from build123d import *
from OCP.BRepFilletAPI import BRepFilletAPI_MakeChamfer

# Parameters (mm, degrees)
BOSS_EXTRUDE1_DEPTH = 15
CUT_EXTRUDE4_DEPTH  = 5
SKETCH7_R           = 3.1
CUT_EXTRUDE6_DEPTH  = 66.86721491
FILLET1_R           = 7.5
CUT_EXTRUDE7_DEPTH  = 5
CUT_EXTRUDE8_DEPTH  = 5
FILLET2_R           = 1.5
BOSS_EXTRUDE2_DEPTH = 5
SKETCH6_R           = 3.1
CUT_EXTRUDE5_DEPTH  = 66.86721491
CHAMFER8_SIZE       = 15
CHAMFER8_SIZE_2     = 5


with BuildPart() as part:
    # Sketch1 → Boss-Extrude1 (new body)
    with BuildSketch(Plane(origin=(0, 0, 0), x_dir=(1, 0, 0), z_dir=(0, 1, 0))):
        Polygon((0, 0), (-35, 0), (-45, 12.85), (-45, 32.85), (-35, 45.7), (0, 45.7), (0, 40.7), (-22.5, 40.7), (-22.5, 35.5), (0, 35.5), (0, 27.85), (-22.5, 27.85), (-22.5, 17.85), (0, 17.85), (0, 10.2), (-22.5, 10.2), (-22.5, 5), (0, 5), align=None)
    extrude(amount=BOSS_EXTRUDE1_DEPTH)

    # Sketch5 → Cut-Extrude4 (cut)
    with BuildSketch(Plane(origin=(0, 15, 0), x_dir=(1, 0, 0), z_dir=(0, 1, 0))):
        Polygon((-41.639528096, 22.85), (-38.319764048, 17.1), (-31.680235952, 17.1), (-28.360471904, 22.85), (-31.680235952, 28.6), (-38.319764048, 28.6), align=None)
    extrude(amount=-CUT_EXTRUDE4_DEPTH, mode=Mode.SUBTRACT)

    # Sketch7 → Cut-Extrude6 (cut, through all)
    with BuildSketch(Plane.XY):
        with Locations((-7.5, 7.5)):
            Circle(SKETCH7_R)
    extrude(amount=-CUT_EXTRUDE6_DEPTH, mode=Mode.SUBTRACT)

    # Fillet1
    fillet1_edges = [part.edges().sort_by_distance(p)[0] for p in [
        (0, 0, -43.2),
        (0, 0, -31.675),
        (0, 0, -2.5),
        (0, 15, -43.2),
        (0, 15, -31.675),
        (0, 15, -2.5),
        (0, 0, -14.025),
        (0, 15, -14.025),
    ]]
    fillet(fillet1_edges, radius=FILLET1_R - 0.0001)  # a hair under: the kernel refuses the full size

    # Sketch8 → Cut-Extrude7 (cut)
    with BuildSketch(Plane.XY.offset(-27.85)):
        Polygon((-9.839641819, 13.713647036), (-14.050997093, 8.580634267), (-11.711355274, 2.366987231), (-5.160358181, 1.286352964), (-0.949002907, 6.419365733), (-3.288644726, 12.633012769), align=None)
    extrude(amount=-CUT_EXTRUDE7_DEPTH, mode=Mode.SUBTRACT)

    # Sketch9 → Cut-Extrude8 (cut)
    with BuildSketch(Plane(origin=(0, 0, -17.85), x_dir=(-1, 0, 0), z_dir=(0, 0, -1))):
        Polygon((9.839641819, 13.713647036), (3.288644726, 12.633012769), (0.949002907, 6.419365733), (5.160358181, 1.286352964), (11.711355274, 2.366987231), (14.050997093, 8.580634267), align=None)
    extrude(amount=-CUT_EXTRUDE8_DEPTH, mode=Mode.SUBTRACT)

    # Fillet2
    fillet2_edges = [part.edges().sort_by_distance(p)[0] for p in [
        (-22.5, 7.5, -40.7),
        (-22.5, 7.5, -35.5),
        (-22.5, 7.5, -27.85),
        (-22.5, 7.5, -17.85),
        (-22.5, 7.5, -10.2),
        (-22.5, 7.5, -5),
    ]]
    fillet(fillet2_edges, radius=FILLET2_R)

    # Sketch15 → Boss-Extrude2 (add)
    with BuildSketch(Plane.XZ):
        Polygon((-35, 0), (-45, -12.85), (-45, -32.85), (-35, -45.7), (-22.5, -45.7), (-22.5, 0), align=None)
    extrude(amount=BOSS_EXTRUDE2_DEPTH)

    # Sketch6 → Cut-Extrude5 (cut, through all)
    with BuildSketch(Plane(origin=(0, 10, 0), x_dir=(1, 0, 0), z_dir=(0, 1, 0))):
        with Locations(Location((-35, 22.85, 0), (0, 0, 270))):
            Circle(SKETCH6_R)
    extrude(amount=-CUT_EXTRUDE5_DEPTH, mode=Mode.SUBTRACT)

    # Chamfer8
    chamfer8_edges_1 = [part.edges().sort_by_distance(p)[0] for p in [
        (-22.5, 0, -3.25),
    ]]
    chamfer8_side_1 = [part.faces().sort_by_distance(p)[0] for p in [
        (-22.4, 0, -3.25),
    ]]
    chamfer8_edges_2 = [part.edges().sort_by_distance(p)[0] for p in [
        (-22.5, 0, -42.45),
    ]]
    chamfer8_side_2 = [part.faces().sort_by_distance(p)[0] for p in [
        (-22.5, -0.1, -42.45),
    ]]
    chamfer8_edges_3 = [part.edges().sort_by_distance(p)[0] for p in [
        (-22.5, 0, -14.025),
    ]]
    chamfer8_side_3 = [part.faces().sort_by_distance(p)[0] for p in [
        (-22.5, -0.1, -14.025),
    ]]
    chamfer8_edges_4 = [part.edges().sort_by_distance(p)[0] for p in [
        (-22.5, 0, -31.675),
    ]]
    chamfer8_side_4 = [part.faces().sort_by_distance(p)[0] for p in [
        (-22.5, -0.1, -31.675),
    ]]
    chamfer8 = BRepFilletAPI_MakeChamfer(part.part.solid().wrapped)
    for e in chamfer8_edges_1:
        chamfer8.Add(CHAMFER8_SIZE - 0.0001, CHAMFER8_SIZE_2 - 0.0001, e.wrapped, chamfer8_side_1[0].wrapped)
    for e in chamfer8_edges_2:
        chamfer8.Add(CHAMFER8_SIZE_2 - 0.0001, CHAMFER8_SIZE - 0.0001, e.wrapped, chamfer8_side_2[0].wrapped)
    for e in chamfer8_edges_3:
        chamfer8.Add(CHAMFER8_SIZE_2 - 0.0001, CHAMFER8_SIZE - 0.0001, e.wrapped, chamfer8_side_3[0].wrapped)
    for e in chamfer8_edges_4:
        chamfer8.Add(CHAMFER8_SIZE_2 - 0.0001, CHAMFER8_SIZE - 0.0001, e.wrapped, chamfer8_side_4[0].wrapped)
    add(Compound.cast(chamfer8.Shape()), mode=Mode.REPLACE)  # a hair under: the kernel refuses the full size


solid = part.part
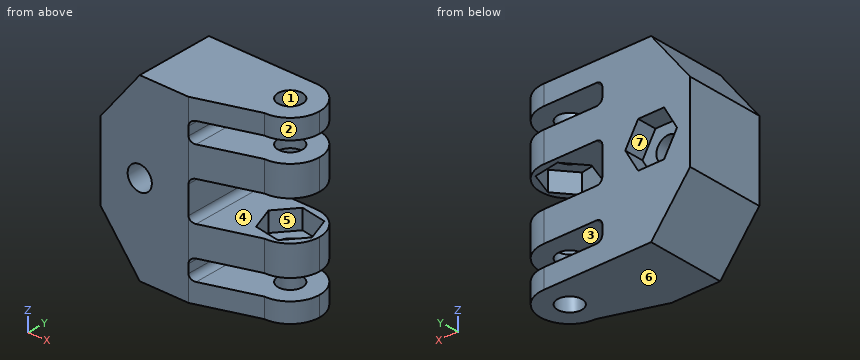
Read the model definition and answer for the solid it produces. Units are mm, in the model's axes. Face numbers are marked on the shaded views. A direction names the side the tool comes from. Coordinates: 2 decimals unless noted, no trailing zeros. Order: outer loops, then holes, each group sorted by start corner. A loop starts at its lowest first (then second) coordinate and runs counter-clockwise, first axis right, second up. Notation, with made-up numbers: M 30,-19 L 72,-19 A24 cw 72,-8 Z; hole C 23.5,80 d10. An arc over 180 degrees is marked long. Put each result on its own line as item: value. Start each with the question number.
Item 1: Section B-B, the plane x = -20 is taken. Determine the outline of the cut face in (y, z).
Item 2: Section C-C, the plane z = -23.5 is taken. Determine the outline of the cut face in (x, y).
Item 3: Consider probe 1 along Z at (x, y) = (-19.5, 13.75); probe 2 along Z at (x, y) = (-4, 3.75); probe 3 along Y at (x, z) = (-7.5, -2.4). Determine where each line is inside the solid, lowest interval first. Write a range as [from, to].
Item 4: Given pin 1 Ø10 at (x, y) = (-7.5, 7.5) entering from +Z; pin 2 Ø3 at (x, y) = (-40.5, 7.5) entering from -Z; pin 3 Ø5 at (y, z) = (-0.5, -24.5) entering from +X; pin 4 Ø10 at (y, z) = (1, -17.5) entering from +X, each flat-ended and moving along its own axis, determine where each tip first touches the part or whether it passes through.
Item 5: The mould has two halves that part along X. Classify the marked faces 1, 2 and 3: +X half, -X half, draft (parallel to the pull), parting line (faces both ways), or undercut.
Item 6: For the marked faces 4, 5, 6 and 7, determine the directions among +Z, -Z, +X, -X, +Y, -Y from which every point of the face is accessible in a straight line to the end or side of a thin tool.
Computed:
1. outline: M -4.17,-45.7 L 15,-45.7 L 15,-40.7 L -4.17,-40.7 Z; M -4.17,-35.5 L 15,-35.5 L 15,-27.85 L -4.17,-27.85 Z; M -4.17,-17.85 L 15,-17.85 L 15,-10.2 L -4.17,-10.2 Z; M -4.17,-5 L 15,-5 L 15,0 L -4.17,0 Z
2. outline: M -45,-5 L -38.03,-5 L -38.03,10 L -41.26,10 L -41.26,15 L -45,15 Z; M -31.97,-5 L -22.5,-5 L -22.5,15 L -28.74,15 L -28.74,10 L -31.97,10 Z
3. probe 1: z = [-45.7, -40.7], [-35.5, -27.85], [-17.85, -10.2], [-5, 0]
3. probe 2: z = [-45.7, -40.7], [-35.5, -32.85], [-12.85, -10.2], [-5, 0]
3. probe 3: y = [0, 4.4], [10.6, 15]
4. pin 1: stops at z = 0
4. pin 2: stops at z = -40.56
4. pin 3: stops at x = -22.35
4. pin 4: stops at x = -0.15
5. face 1: undercut
5. face 2: +X half
5. face 3: draft
6. face 4: +X, +Y, -Y
6. face 5: none
6. face 6: -Z, +X, -X, +Y, -Y
6. face 7: +Y
